from build123d import *

# Parameters (mm, degrees)
BOSS_EXTRUDE1_DEPTH = 4
SKETCH2_W           = 7
SKETCH2_H           = 16
BOSS_EXTRUDE2_DEPTH = 8
SKETCH3_W           = 13.452288764
SKETCH3_H           = 8.193666793
BOSS_EXTRUDE3_DEPTH = 4.698
FILLET1_R           = 1.27
SKETCH4_R           = 1.5
CUT_EXTRUDE1_DEPTH  = 5


with BuildPart() as part:
    # Sketch1 → Boss-Extrude1 (new body)
    with BuildSketch(Plane(origin=(0, 0, 0), x_dir=(1, 0, 0), z_dir=(0, 1, 0))):
        with BuildLine():
            Line((-19.96, -10.5), (19.96, -10.5))
            ThreePointArc((19.96, -10.5), (21.756051224, -9.756051224), (22.5, -7.96))
            Line((22.5, -7.96), (22.5, 7.96))
            ThreePointArc((22.5, 7.96), (21.756051224, 9.756051224), (19.96, 10.5))
            Line((19.96, 10.5), (-19.96, 10.5))
            ThreePointArc((-19.96, 10.5), (-21.756051224, 9.756051224), (-22.5, 7.96))
            Line((-22.5, 7.96), (-22.5, -7.96))
            ThreePointArc((-22.5, -7.96), (-21.756051224, -9.756051224), (-19.96, -10.5))
        make_face()
    extrude(amount=BOSS_EXTRUDE1_DEPTH)

    # Sketch2 → Boss-Extrude2 (add)
    with BuildSketch(Plane(origin=(0, 4, 0), x_dir=(1, 0, 0), z_dir=(0, 1, 0))):
        with Locations((19, 0)):
            Rectangle(SKETCH2_W, SKETCH2_H)
    extrude(amount=BOSS_EXTRUDE2_DEPTH)

    # Sketch3 → Boss-Extrude3 (add)
    with BuildSketch(Plane(origin=(0, 4, 0), x_dir=(1, 0, 0), z_dir=(0, 1, 0))):
        with Locations((-3.928679787, 3.057338356)):
            Rectangle(SKETCH3_W, SKETCH3_H)
    extrude(amount=BOSS_EXTRUDE3_DEPTH)

    # Fillet1
    fillet1_edges = [part.edges().sort_by_distance(p)[0] for p in [
        (-3.928679787, 8.698, 1.039495041),
        (-3.928679787, 8.698, -7.154171752),
    ]]
    fillet(fillet1_edges, radius=FILLET1_R)

    # Sketch4 → Cut-Extrude1 (cut, through all)
    with BuildSketch(Plane(origin=(0, 4, 0), x_dir=(1, 0, 0), z_dir=(0, 1, 0))):
        with Locations((-18.902, -6.01)):
            Circle(SKETCH4_R)
        with Locations((10.308, 6.69)):
            Circle(SKETCH4_R)
    extrude(amount=-CUT_EXTRUDE1_DEPTH, mode=Mode.SUBTRACT)


solid = part.part
The model under review builds one solid part; all positions refer to its coordinate system, in mm. A direction names the side the tool comes from. Coordinates: 2 decimals unless noted, no trailing zeros. Order: outer loops, then holes, each group sorted by start corner. A loop starts at its lowest first (then second) coordinate and runs counter-clockwise, first axis right, second up. Notation, with made-up numbers: (-7, 17) -> (43, 17) arc R11 ccw to (43, 35) -> close; hole circle Ø11 at (70.25, 10.5). An arc over 180 degrees is marked (long way). Answer in a Markdown table with one row per item.
(1) Consider section D-D (x = -10). Write out the cut boundary in (y, z).
Answers:
| item | result |
|---|---|
| outline | (0, -10.5) -> (4, -10.5) -> (4, -7.15) -> (7.43, -7.15) arc R1.27 ccw to (8.7, -5.88) -> (8.7, -0.23) arc R1.27 ccw to (7.43, 1.04) -> (4, 1.04) -> (4, 10.5) -> (0, 10.5) -> close |
(2) Machinability: for faces 1 (the flat face through (15.5, 8, 0)), 2 (the flat face through (-10.655, 6, -3)), 3 (the flat face through (-4, 6, -7.154)), which of the approach directions +Z, -Z, +X, -X, +Y, -Y give a long, thin tool a straight path to every point of the face, cutting with its end or side? Answer none if there is none.
Answers:
| item | result |
|---|---|
| face 1 | +Z, -Z, +Y |
| face 2 | +Z, -Z, -X, +Y |
| face 3 | -Z, -X, +Y |
(3) Consider section A-A (z = 6.01). Write out the cut boundary in (x, y).
Answers:
| item | result |
|---|---|
| outline | (-22.5, 0) -> (-20.4, 0) -> (-20.4, 4) -> (-22.5, 4) -> close; (-17.4, 0) -> (22.5, 0) -> (22.5, 12) -> (15.5, 12) -> (15.5, 4) -> (-17.4, 4) -> close |
(4) Consider section B-B (y = 4.5). Write out the cut boundary in (x, z), plus the area to 3 significant figures.
Answers:
| item | result |
|---|---|
| outline | (-10.65, -7.15) -> (2.8, -7.15) -> (2.8, 1.04) -> (-10.65, 1.04) -> close; (15.5, -8) -> (22.5, -8) -> (22.5, 8) -> (15.5, 8) -> close |
| area | 222 mm² |
(5) Wall thickness on line 1 along X through (y, z) = (1.3, -6.69); line 2 along X through (y, z) = (3.05, 6.01); line 3 along Y through (x, z) = (17, -9.5): over which ranges is each line inside the solid? List them lowest first.
Answers:
| item | result |
|---|---|
| line 1 | -22.5 to 8.81, 11.81 to 22.5 |
| line 2 | -22.5 to -20.4, -17.4 to 22.5 |
| line 3 | 0 to 4 |
(6) Insertion check: pin 1 (2.5 mm diameter, centred on x = -7, y = 6.5, fed in from -Z); pin 2 (1 mm diameter, centred on x = 17.5, y = 7.5, fed in from +Z); pin 3 (2 mm diameter, centred on x = 0, z = 5.5, fed in from +Y). Each pin has a flat end and moves straight along its axis. Give the tip position at first contact, or say it passes through.
Answers:
| item | result |
|---|---|
| pin 1 | z = -7.15 |
| pin 2 | z = 8 |
| pin 3 | y = 4 |
(7) The part is to be moulded in two halves that separate along X. For faces 4 (the cylindrical face through (-21.736, 1.972, -9.776)), 5 (the flat face through (22.5, 6, 0)), 6 (the flat face through (0, 4, 2)), say which applies: +X half, -X half, draft (parallel to the pull), parting line (faces both ways), or undercut.
Answers:
| item | result |
|---|---|
| face 4 | -X half |
| face 5 | +X half |
| face 6 | undercut |
(8) Consider section C-C (y = 2). Write out the cut boundary in (x, z), plus the area to 3 significant figures.
Answers:
| item | result |
|---|---|
| outline | (-22.5, -7.96) arc R2.54 ccw to (-19.96, -10.5) -> (19.96, -10.5) arc R2.54 ccw to (22.5, -7.96) -> (22.5, 7.96) arc R2.54 ccw to (19.96, 10.5) -> (-19.96, 10.5) arc R2.54 ccw to (-22.5, 7.96) -> close; hole circle Ø3 at (-18.9, 6.01); hole circle Ø3 at (10.31, -6.69) |
| area | 925 mm² |
